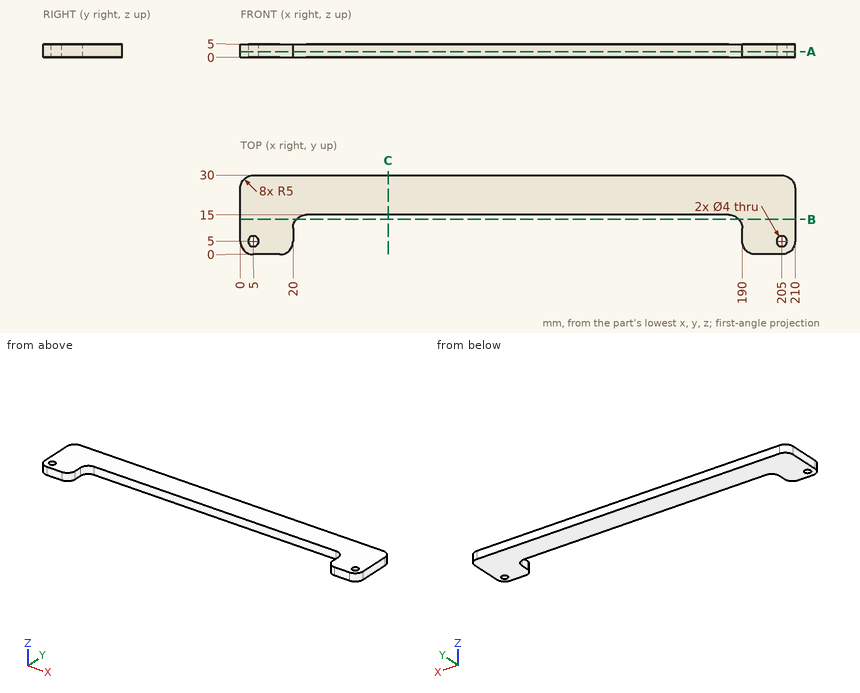
Can you work these out from the drawing? Everything is in mm from the part's minimum corner. Give positions to 0.01 mm unless a question says otherwise; leave off trailing zeros. Order: outer loops, then holes, each group sorted by start corner. A loop starts at its lowest first (then second) coordinate and runs counter-clockwise, first axis right, second up.
1. Suppose I cut it at C-C (x = 56). List the corners of the cut face in (y, z) for me.
2. Suppose I cut it at A-A (z = 2.1). List the corners of the cut face in (x, y) for me.
3. I need wall thicknesses on L1, parallel to Y at x = 5, z = 3.85; L2, parallel to X at y = 4, z = 3.75; L3, parallel to Y at x = 117, z = 4.85. Which ranges of each line are inside material? Lowest first, please.
4. Suppose I cut it at B-B (y = 13.25). List the corners of the cut face in (x, z) for me.
Solved:
1. outline: (15, 0) - (30, 0) - (30, 5) - (15, 5) - close
2. outline: (0, 5) arc R5 ccw to (5, 0) - (15, 0) arc R5 ccw to (20, 5) - (20, 10) arc R5 cw to (25, 15) - (185, 15) arc R5 cw to (190, 10) - (190, 5) arc R5 ccw to (195, 0) - (205, 0) arc R5 ccw to (210, 5) - (210, 25) arc R5 ccw to (205, 30) - (5, 30) arc R5 ccw to (0, 25) - close; hole circle Ø4 at (5, 5); hole circle Ø4 at (205, 5)
3. L1: y = 0 to 3, 7 to 30
3. L2: x = 0.1 to 3.27, 6.73 to 19.9, 190.1 to 203.27, 206.73 to 209.9
3. L3: y = 15 to 30
4. outline: (0, 0) - (21.2, 0) - (21.2, 5) - (0, 5) - close; (188.8, 0) - (210, 0) - (210, 5) - (188.8, 5) - close
